from build123d import *

# Parameters (mm, degrees)
SKETCH_2_W          = 30
SKETCH_2_H          = 60
EXTRUDE_1_DEPTH     = 4
SKETCH_3_R          = 4.195093659
CUT_EXTRUDE_1_DEPTH = 34.778691508
FILLET_1_R          = 10


with BuildPart() as part:
    # 草圖2 → 填料-伸長1 (new body)
    with BuildSketch(Plane.XY):
        Rectangle(SKETCH_2_W, SKETCH_2_H)
    extrude(amount=EXTRUDE_1_DEPTH)

    # 草圖3 → 除料-伸長1 (cut, through all)
    with BuildSketch(Plane.XY.offset(4)):
        with Locations((5, 15)):
            Circle(SKETCH_3_R)
    extrude(amount=-CUT_EXTRUDE_1_DEPTH, mode=Mode.SUBTRACT)

    # 圓角1
    fillet_1_edges = [part.edges().sort_by_distance(p)[0] for p in [
        (-15, 30, 2),
        (15, 30, 2),
        (15, -30, 2),
        (-15, -30, 2),
    ]]
    fillet(fillet_1_edges, radius=FILLET_1_R)


solid = part.part
Model file for the job. Use its own axes, mm. Coordinates: 2 decimals unless noted, no trailing zeros. Write each loop counter-clockwise with the first axis right and the second up, starting at its lowest first coordinate (ties: lowest second). Pieces come first, ordered by that corner, then holes. Notation, with made-up numbers: (17.5, -1.5) - (39.5, -1.5) arc R21 cw to (39.5, 19.5) - close; hole circle Ø5 at (78.25, 83). An arc over 180 degrees is marked (long way). Write each question's results on one line, items separated by ' | '. Start each with the question number.
1) Cut at B-B (z = 2.7). Write the cut outline in (x, y).
2) Flat gauge pins, fed straight in: P1, Ø2, axis at x = 6.5, z = 0.5, coming from the -Y side; P2, Ø10, axis at x = 11, y = 15, coming from the -Z side; P3, Ø5, axis at x = 5, y = 15, coming from the +Z side. Where does each tip first touch, or does it go through?
3) Cut at D-D (y = -26). Write the cut outline in (x, z), then the cut area to 3 significant figures.
4) Cut at A-A (x = 6). Write the cut outline in (y, z).
5) Probe line 1 along X through (y, z) = (12.5, 3.65); line 2 along X through (y, z) = (14.5, 1.25); line 3 along Y through (x, z) = (10.5, 2.35). List the from-to ranges inside material, lowest first. Write a range as from..to.
6) Cut at C-C (y = 15). Write the cut outline in (x, z), then the cut area to 3 significant figures.
7) Mould opens along X. For faces 1 (the face through (-12.15, 26.99, 2.03)), 2 (the face through (15, 0, 2)), 3 (the face through (0, 0, 0)), 4 (the face through (4.45, 19.16, 2.03)) say: pulls with the +X half, pulls with the -X half, needs draft (parallel to the pull), parting line crosses it, or undercut.
Returned:
1) outline: (-15, -20) arc R10 ccw to (-5, -30) - (5, -30) arc R10 ccw to (15, -20) - (15, 20) arc R10 ccw to (5, 30) - (-5, 30) arc R10 ccw to (-15, 20) - close; hole circle Ø8.39 at (5, 15)
2) P1: y = -29.99 | P2: z = 0 | P3: through
3) outline: (-13, 0) - (13, 0) - (13, 4) - (-13, 4) - close | area: 104 mm^2
4) outline: (-29.95, 0) - (10.93, 0) - (10.93, 4) - (-29.95, 4) - close; (19.07, 0) - (29.95, 0) - (29.95, 4) - (19.07, 4) - close
5) line 1: -15..1.63, 8.37..15 | line 2: -15..0.83, 9.17..15 | line 3: -28.35..28.35
6) outline: (-15, 0) - (0.8, 0) - (0.8, 4) - (-15, 4) - close; (9.2, 0) - (15, 0) - (15, 4) - (9.2, 4) - close | area: 86.4 mm^2
7) face 1: pulls with the -X half | face 2: pulls with the +X half | face 3: needs draft | face 4: undercut
